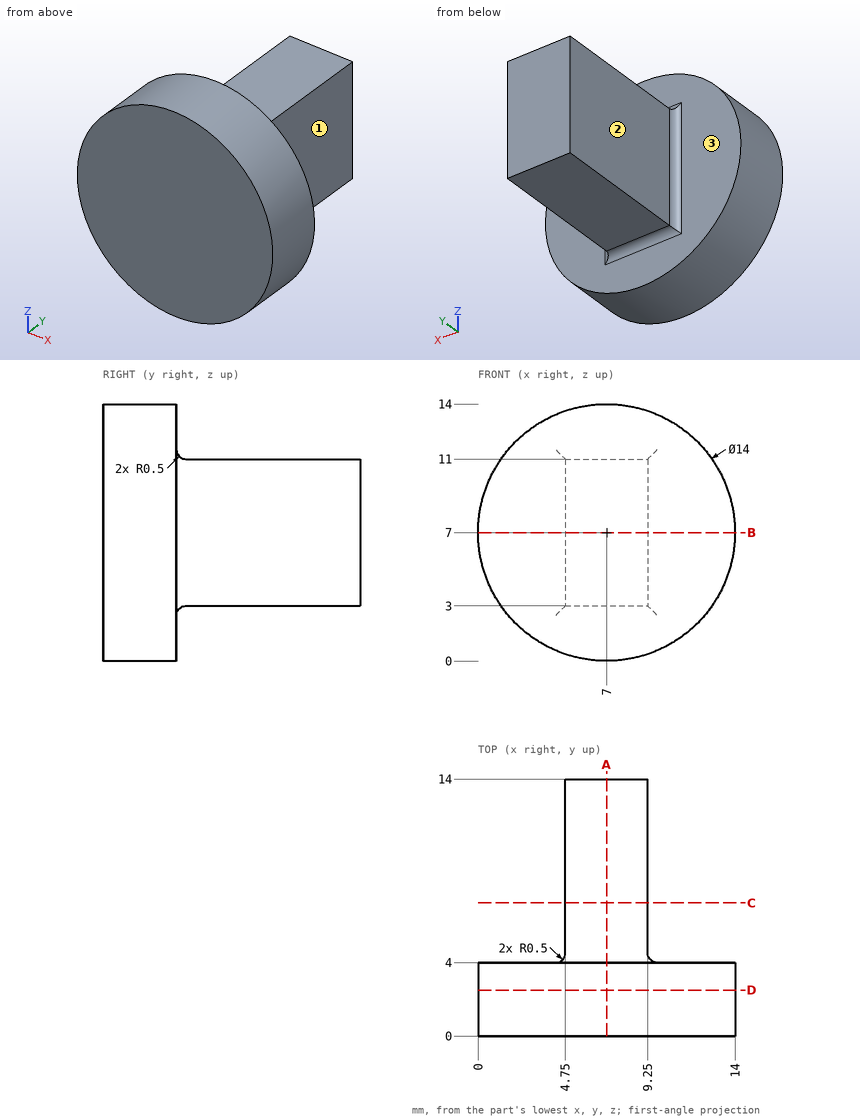
Design review of the part shown in the three views and the two pictorial views. Dimensions are in mm from the part's minimum x, y and z. A direction names the side the tool comes from. Give positions to 0.01 mm unless a question says otherwise; leave off trailing zeros. Order: outer loops, then holes, each group sorted by start corner. A loop starts at its lowest first (then second) coordinate and runs counter-clockwise, first axis right, second up. Notation, with made-up numbers: M 29,56 L 42,56 A13 cw 42,77 Z; hole C -1.75,89.5 d7. An arc over 180 degrees is marked long. Answer in a Markdown table with one row per item. Add a question column.
(1) For the marked faces 1, 2 and 3, list the 3-axis set-ups (+Z, -Z, +X, -X, +Y, -Y) from which the entire face can be reached by the end or side of a thin tool; tool diameter is ignored.
(2) For pin 1 (4 mm diameter, centred on y = 7.5, z = 8.5, fed in from +X); pin 2 (6 mm diameter, centred on y = 6.5, z = 10.5, fed in from -X); pin 3 (2 mm diameter, centred on x = 6.5, y = 11, fed in from -Z), all flat-tipped, find the tip position at first contact; note any pin that passes through.
(3) Consider section A-A on x = 7. State the section outline as (y, z) points, and give its area (3 significant figures).
(4) Consider section C-C on y = 7.25. State the section outline as (x, z) points, and give its area (3 significant figures).
(5) Consider section D-D on y = 2.5. State the section outline as (x, z) points.
(6) Wall thickness on probe 1 along Y at (x, z) = (4, 2); probe 2 along Z at (x, y) = (6.75, 10.5); probe 3 along X at (y, z) = (10.75, 6.5): over which ranges is each line inside the solid? List them lowest first. Write a range as [from, to].
(7) Consider section B-B on z = 7. State the section outline as (x, y) points, and give its area (3 significant figures).
Evaluation:
| question | item | result |
|---|---|---|
| 1 | face 1 | +Z, -Z, +X, +Y |
| 1 | face 2 | +Z, -Z, -X, +Y |
| 1 | face 3 | +Y |
| 2 | pin 1 | stops at x = 9.25 |
| 2 | pin 2 | stops at x = 0.25 |
| 2 | pin 3 | stops at z = 3 |
| 3 | outline | M 0,0 L 4,0 L 4,2.5 A0.5 cw 4.5,3 L 14,3 L 14,11 L 4.5,11 A0.5 cw 4,11.5 L 4,14 L 0,14 Z |
| 3 | area | 136 mm^2 |
| 4 | outline | M 4.75,3 L 9.25,3 L 9.25,11 L 4.75,11 Z |
| 4 | area | 36.0 mm^2 |
| 5 | outline | C 7,7 d14 |
| 6 | probe 1 | y = [0, 4] |
| 6 | probe 2 | z = [3, 11] |
| 6 | probe 3 | x = [4.75, 9.25] |
| 7 | outline | M 0,0 L 14,0 L 14,4 L 9.75,4 A0.5 cw 9.25,4.5 L 9.25,14 L 4.75,14 L 4.75,4.5 A0.5 cw 4.25,4 L 0,4 Z |
| 7 | area | 101 mm^2 |
